Design review of the part built by this model. Coordinates are the model's own, in mm. Coordinates: 2 decimals unless noted, no trailing zeros. Loops run counter-clockwise (first coordinate to the right, second up) from the corner with the lowest first, then second, coordinate; pieces in that order, holes last. Notation, with made-up numbers: (30, -9.75) - (49, -9.75) arc R26 cw to (49, 14.25) - close; hole circle Ø1 at (17, 73.5). An arc over 180 degrees is marked (long way). One line per question, with ' | ' between items.
from build123d import *

# Parameters (mm, degrees)
SKETCH2_R                = 27.94
BOSS_EXTRUDE1_DEPTH      = 5.08
SKETCH3_R                = 22.86
CUT_EXTRUDE1_DEPTH       = 40.838343339
BOSS_EXTRUDE2_DEPTH      = 1.524
BOSS_EXTRUDE2_DEPTH_BACK = 6.604
SKETCH4_R                = 24.638
SKETCH4_R_2              = 22.86
SKETCH5_R                = 8.89
SKETCH5_W                = 5.08
SKETCH5_H                = 18.131594767
SKETCH5_W_2              = 2.51172526
SKETCH5_H_2              = 8.964878854
BOSS_EXTRUDE4_DEPTH      = 5.08
SKETCH6_R                = 4.191
SKETCH6_R_2              = 2.667
BOSS_EXTRUDE5_DEPTH      = 0.762
CUT_EXTRUDE2_START       = -2.794
SKETCH8_R                = 2.667
CUT_EXTRUDE2_DEPTH       = 2.794
CUT_EXTRUDE3_DEPTH       = 2.794
SKETCH10_R               = 1.1176
CUT_EXTRUDE4_DEPTH       = 40.776756831
SKETCH11_R               = 1.016
CUT_EXTRUDE5_DEPTH       = 41.061203377


with BuildPart() as part:
    # Sketch2 → Boss-Extrude1 (new body)
    with BuildSketch(Plane(origin=(0, 0, 0), x_dir=(1, 0, 0), z_dir=(0, 1, 0))):
        with Locations(Location((0, 0, 0), (0, 0, 270))):
            Circle(SKETCH2_R)
    extrude(amount=BOSS_EXTRUDE1_DEPTH)

    # Sketch3 → Cut-Extrude1 (cut, through all)
    with BuildSketch(Plane(origin=(0, 5.08, 0), x_dir=(1, 0, 0), z_dir=(0, 1, 0))):
        with Locations(Location((0, 0, 0), (0, 0, 270))):
            Circle(SKETCH3_R)
    extrude(amount=-CUT_EXTRUDE1_DEPTH, mode=Mode.SUBTRACT)

    # Sketch4 → Boss-Extrude2 (add, two sides: drawn at the far end of the back side and taken through both)
    with BuildSketch(Plane(origin=(0, 5.08, 0), x_dir=(1, 0, 0), z_dir=(0, 1, 0)).offset(-BOSS_EXTRUDE2_DEPTH_BACK)):
        with Locations(Location((0, 0, 0), (0, 0, 270))):
            Circle(SKETCH4_R)
        with Locations(Location((0, 0, 0), (0, 0, 270))):
            Circle(SKETCH4_R_2, mode=Mode.SUBTRACT)
    extrude(amount=BOSS_EXTRUDE2_DEPTH + BOSS_EXTRUDE2_DEPTH_BACK)

    # Sketch5 → Boss-Extrude4 (add)
    # profile 1 of 6: a face of its own
    with BuildSketch(Plane(origin=(0, 5.08, 0), x_dir=(1, 0, 0), z_dir=(0, 1, 0))):
        Circle(SKETCH5_R)
    # profile 2 of 6: a face of its own
    with BuildSketch(Plane(origin=(0, 5.08, 0), x_dir=(1, 0, 0), z_dir=(0, 1, 0))):
        Polygon((5.278203535, 4.385706339), (22.522374889, 9.988677257), (24.092181221, 5.157310154), (6.848009867, -0.445660764), align=None)
        Polygon((10.810222047, 2.19196195), (10.034056257, 4.580754625), (18.560162709, 7.351054544), (19.336328499, 4.962261868), align=None, mode=Mode.SUBTRACT)
    # profile 3 of 6: a face of its own
    with BuildSketch(Plane(origin=(0, 5.08, 0), x_dir=(1, 0, 0), z_dir=(0, 1, 0))):
        with Locations((0, 15.440925042)):
            Rectangle(SKETCH5_W, SKETCH5_H)
        with Locations((0, 15.440925041)):
            Rectangle(SKETCH5_W_2, SKETCH5_H_2, mode=Mode.SUBTRACT)
    # profile 4 of 6: a face of its own
    with BuildSketch(Plane(origin=(0, 5.08, 0), x_dir=(1, 0, 0), z_dir=(0, 1, 0))):
        Polygon((5.802109184, -3.664612076), (16.459593189, -18.333380377), (12.349786858, -21.319329459), (1.692302853, -6.650561157), align=None)
        Polygon((5.425222021, -9.603778627), (7.457250442, -8.127423562), (12.726674021, -15.380162907), (10.6946456, -16.856517973), align=None, mode=Mode.SUBTRACT)
    # profile 5 of 6: a face of its own
    with BuildSketch(Plane(origin=(0, 5.08, 0), x_dir=(1, 0, 0), z_dir=(0, 1, 0))):
        Polygon((-1.692302853, -6.650561157), (-12.349786858, -21.319329459), (-16.459593189, -18.333380377), (-5.802109184, -3.664612076), align=None)
        Polygon((-7.457250442, -8.127423562), (-5.425222021, -9.603778627), (-10.6946456, -16.856517973), (-12.726674021, -15.380162907), align=None, mode=Mode.SUBTRACT)
    # profile 6 of 6: a face of its own
    with BuildSketch(Plane(origin=(0, 5.08, 0), x_dir=(1, 0, 0), z_dir=(0, 1, 0))):
        Polygon((-6.848009867, -0.445660764), (-24.092181221, 5.157310154), (-22.522374889, 9.988677257), (-5.278203535, 4.385706339), align=None)
        Polygon((-10.034056257, 4.580754625), (-10.810222047, 2.19196195), (-19.336328499, 4.962261868), (-18.560162709, 7.351054544), align=None, mode=Mode.SUBTRACT)
    extrude(amount=-BOSS_EXTRUDE4_DEPTH)

    # Sketch6 → Boss-Extrude5 (add)
    with BuildSketch(Plane(origin=(0, 5.08, 0), x_dir=(1, 0, 0), z_dir=(0, 1, 0))):
        with Locations(Location((0, 0, 0), (0, 0, 90))):
            Circle(SKETCH6_R)
        with Locations(Location((0, 0, 0), (0, 0, 90))):
            Circle(SKETCH6_R_2, mode=Mode.SUBTRACT)
    extrude(amount=BOSS_EXTRUDE5_DEPTH)

    # Sketch8 → Cut-Extrude2 (cut)
    with BuildSketch(Plane(origin=(0, 5.842, 0), x_dir=(1, 0, 0), z_dir=(0, 1, 0)).offset(CUT_EXTRUDE2_START)):
        with Locations(Location((0, 0, 0), (0, 0, 90))):
            Circle(SKETCH8_R)
    extrude(amount=CUT_EXTRUDE2_DEPTH, mode=Mode.SUBTRACT)

    # Sketch9 → Cut-Extrude3 (cut)
    with BuildSketch(Plane(origin=(0, 5.842, 0), x_dir=(1, 0, 0), z_dir=(0, 1, 0))):
        Polygon((0, 3.125091392), (-0.334263734, 2.645969908), (-0.777178626, 3.026910899), (-0.981788182, 2.479713888), (-1.50552426, 2.738538463), (-1.567623268, 2.157648324), (-2.139272268, 2.278093583), (-2.054958818, 1.700009781), (-2.638601932, 1.674507705), (-2.413173749, 1.135553371), (-2.972138533, 0.965706349), (-2.619760098, 0.499745966), (-3.118924738, 0.196226112), (-2.661737285, -0.167462316), (-3.069737432, -0.585583733), (-2.536467729, -0.824148324), (-2.827667233, -1.330599199), (-2.251822577, -1.429050062), (-2.407924303, -1.992008224), (-1.825687132, -1.944159329), (-1.836882632, -2.528252045), (-1.284837049, -2.337109916), (-1.150422871, -2.905636493), (-0.663255929, -2.583211291), (-0.391677809, -3.100449113), (0, -2.667), (0.391677809, -3.100449113), (0.663255929, -2.583211291), (1.150422871, -2.905636493), (1.284837049, -2.337109916), (1.836882632, -2.528252045), (1.825687132, -1.944159329), (2.407924303, -1.992008224), (2.251822577, -1.429050062), (2.827667233, -1.330599199), (2.536467729, -0.824148324), (3.069737432, -0.585583733), (2.661737285, -0.167462316), (3.118924738, 0.196226112), (2.619760098, 0.499745966), (2.972138533, 0.965706349), (2.413173749, 1.135553371), (2.638601932, 1.674507705), (2.054958818, 1.700009781), (2.139272268, 2.278093583), (1.567623268, 2.157648324), (1.50552426, 2.738538463), (0.981788182, 2.479713888), (0.777178626, 3.026910899), (0.334263734, 2.645969908), align=None)
    extrude(amount=-CUT_EXTRUDE3_DEPTH, mode=Mode.SUBTRACT)

    # Sketch10 → Cut-Extrude4 (cut, through all)
    with BuildSketch(Plane(origin=(0, 3.048, 0), x_dir=(1, 0, 0), z_dir=(0, 1, 0))):
        with Locations(Location((0, 0, 0), (0, 0, 270))):
            Circle(SKETCH10_R)
    extrude(amount=-CUT_EXTRUDE4_DEPTH, mode=Mode.SUBTRACT)

    # Sketch11 → Cut-Extrude5 (cut, through all)
    with BuildSketch(Plane(origin=(0, 5.08, 0), x_dir=(1, 0, 0), z_dir=(0, 1, 0))):
        with Locations(Location((0, 6.5405, 0), (0, 0, 270))):
            Circle(SKETCH11_R)
        with Locations(Location((6.5405, 0, 0), (0, 0, 270))):
            Circle(SKETCH11_R)
        with Locations(Location((0, -6.5405, 0), (0, 0, 270))):
            Circle(SKETCH11_R)
        with Locations(Location((-6.5405, 0, 0), (0, 0, 270))):
            Circle(SKETCH11_R)
    extrude(amount=-CUT_EXTRUDE5_DEPTH, mode=Mode.SUBTRACT)


solid = part.part
Q1. Take a section at A-A (x = 13.5). Give the boundary of the cut face in (y, z), plus the area to 3 significant figures.
Returned:
outline: (-1.52, -20.61) - (0, -20.61) - (0, -24.46) - (5.08, -24.46) - (5.08, -20.61) - (6.6, -20.61) - (6.6, -18.45) - (-1.52, -18.45) - close; (-1.52, 18.45) - (0, 18.45) - (0, 14.26) - (5.08, 14.26) - (5.08, 18.45) - (6.6, 18.45) - (6.6, 20.61) - (5.08, 20.61) - (5.08, 24.46) - (0, 24.46) - (0, 20.61) - (-1.52, 20.61) - close; (0, -7.06) - (5.08, -7.06) - (5.08, -5.71) - (0, -5.71) - close; (0, -3.07) - (5.08, -3.07) - (5.08, -1.72) - (0, -1.72) - close | area: 109 mm²
Q2. For pin 1 (4 mm diameter, centred on y = 2, z = -12.5, fed in from +X); pin 2 (1.8 mm diameter, centred on x = 0, z = 6.54, fed in from -Y); pin 3 (1.5 mm diameter, centred on x = 15.5, y = 1.5, fed in from -Z); pin 4 (21.5 mm diameter, centred on x = -4.5, z = -5.5, fed in from +Y), all flat-tipped, find the tip position at first contact; note any pin that passes through.
Returned:
pin 1: stops at x = 25.89 | pin 2: passes through | pin 3: stops at z = -23.73 | pin 4: stops at y = 5.84
Q3. Take a section at D-D (x = 25.5). Give the boundary of the cut face in (y, z), plus the area to 3 significant figures.
Returned:
outline: (0, -11.42) - (5.08, -11.42) - (5.08, 11.42) - (0, 11.42) - close | area: 116 mm²
Q4. To check wall thickness, follow line 1 along X through (y, z) = (3, 0); line 2 along X through (y, z) = (0.75, 14.5); line 3 along Z through (x, y) = (12, 0.75). State the ranges of each line that lie inside material, in increasing order.
Returned:
line 1: x = -27.94 to -22.86, -8.89 to -7.56, -5.52 to -1.12, 1.12 to 5.52, 7.56 to 8.89, 22.86 to 27.94 | line 2: x = -23.88 to -17.67, -13.67 to -12.09, -8.98 to -7.4, 7.4 to 8.98, 12.09 to 13.67, 17.67 to 23.88 | line 3: z = -25.23 to -19.46, -6.57 to -5.22, -2.58 to -1.23, 12.2 to 14.38, 15.91 to 25.23
Q5. Take a section at B-B (z = 13). State how many separate pieces and enclosed holes the cut face has, plus the area to 3 significant figures.
Returned:
separate pieces: 6 | enclosed holes: 0 | area: 105 mm²
